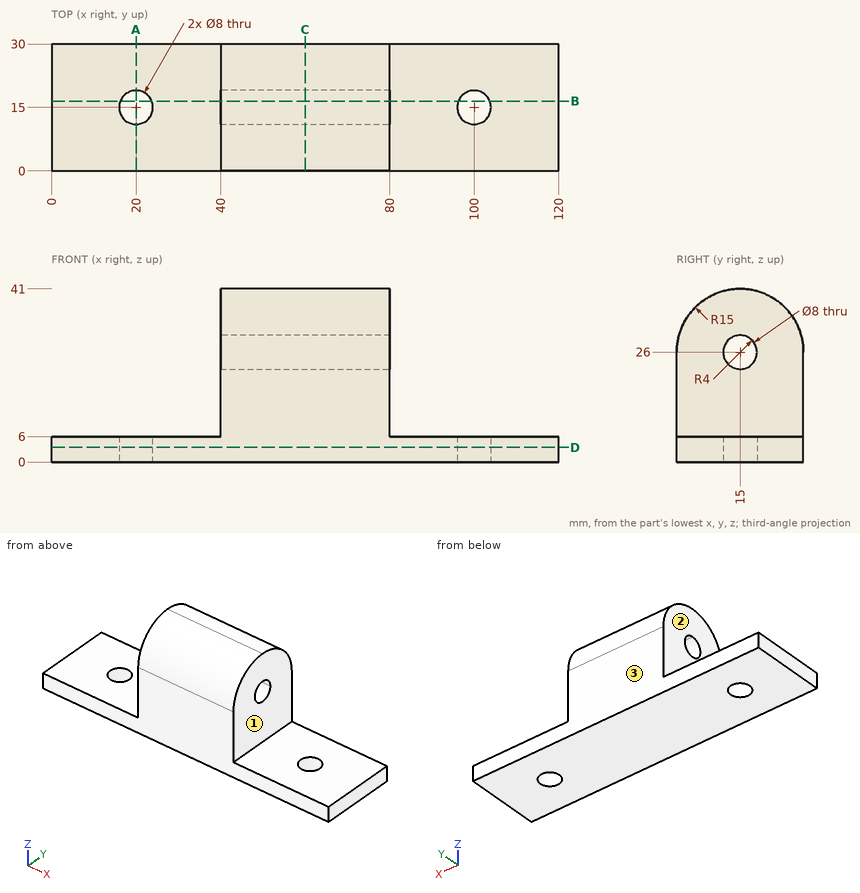
Study the drawing (mm; zero at the part's minimum x, y, z) and answer. A direction names the side the tool comes from. Give positions to 0.01 mm unless a question says otherwise; leave off trailing zeros. Loops run counter-clockwise (first coordinate to the right, second up) from the corner with the lowest first, then second, coordinate; pieces in that order, holes last. Notation, with made-up numbers: (58, 26.5) - (78, 26.5) arc R25 cw to (78, 60.5) - close; hole circle Ø5 at (19.25, -16.5). An arc over 180 degrees is marked (long way). Return JSON: item names as keys, results as strings. Group by question number.
1. Find section A-A (x = 20). Write down the section's boundary in (y, z), then the cut area to 3 significant figures.
2. Given pin 1 Ø5 at (x, y) = (100, 15) entering from -Z; pin 2 Ø4 at (y, z) = (13.5, 13.5) entering from -X; pin 3 Ø6 at (x, z) = (56.5, 36) entering from +Y; pin 4 Ø5 at (x, y) = (71.5, 5.5) entering from +Z, each flat-ended and moving along its own axis, determine where each tip first touches the part or whether it passes through.
3. Straight lines are drawn through the part: line 1 (Y direction, x = 60, z = 26); line 2 (X direction, y = 24, z = 19); line 3 (Z direction, x = 8.5, y = 5.5). For each, find the intervals that lie inside material, in ascending order. Write a range as [from, to].
4. Find section D-D (z = 3.5). Write down the section's boundary in (x, y), then the cut area to 3 significant figures.
5. Which of the six approach directions +Z, -Z, +X, -X, +Y, -Y give full straight-line access (tool end or side, diameter ignored) to the marked faces 1, 2 and 3?
6. Find section B-B (y = 16.5). Write down the section's boundary in (x, z), then the cut area to 3 significant figures.
7. Find section C-C (x = 60). Write down the section's boundary in (y, z), then the cut area to 3 significant figures.
Verdict:
{
 "1": {"outline": "(0, 0) - (11, 0) - (11, 6) - (0, 6) - close; (19, 0) - (30, 0) - (30, 6) - (19, 6) - close", "area": "132 mm^2"},
 "2": {"pin 1": "passes through", "pin 2": "stops at x = 40", "pin 3": "stops at y = 28.27", "pin 4": "stops at z = 39.27"},
 "3": {"line 1": "y = [0, 11], [19, 30]", "line 2": "x = [40, 80]", "line 3": "z = [0, 6]"},
 "4": {"outline": "(0, 0) - (120, 0) - (120, 30) - (0, 30) - close; hole circle Ø8 at (20, 15); hole circle Ø8 at (100, 15)", "area": "3,500 mm^2"},
 "5": {"face 1": "+Z, +X, +Y, -Y", "face 2": "+Z, -X, +Y, -Y", "face 3": "+Z, -Z, +X, -X, +Y"},
 "6": {"outline": "(0, 0) - (16.29, 0) - (16.29, 6) - (0, 6) - close; (23.71, 0) - (96.29, 0) - (96.29, 6) - (80, 6) - (80, 22.29) - (40, 22.29) - (40, 6) - (23.71, 6) - close; (40, 29.71) - (80, 29.71) - (80, 40.92) - (40, 40.92) - close; (103.71, 0) - (120, 0) - (120, 6) - (103.71, 6) - close", "area": "1,730 mm^2"},
 "7": {"outline": "(0, 0) - (30, 0) - (30, 26) arc R15 ccw to (15, 41) arc R15 ccw to (0, 26) - close; hole circle Ø8 at (15, 26)", "area": "1,080 mm^2"}
}
